```python
from build123d import *

# Parameters (mm, degrees)
SKETCH1_W           = 13
SKETCH1_H           = 1
SKETCH1_W_2         = 15
BOSS_EXTRUDE1_DEPTH = 6
BOSS_EXTRUDE2_DEPTH = 1


with BuildPart() as part:
    # Sketch1 → Boss-Extrude1 (new body)
    with BuildSketch(Plane(origin=(0, 0, 0), x_dir=(1, 0, 0), z_dir=(0, 1, 0))):
        with Locations((-9.5, 2.5)):
            Rectangle(SKETCH1_W, SKETCH1_H)
        Polygon((-17, 0), (-16, 0), (-16, 1), (-16, 2), (-16, 3), (-17, 3), align=None)
        with Locations((-8.5, 0.5)):
            Rectangle(SKETCH1_W_2, SKETCH1_H)
        Polygon((-1, 0), (0, 0), (0, 3), (-1, 3), (-1, 1), align=None)
    extrude(amount=BOSS_EXTRUDE1_DEPTH)

    # Sketch1_3 → Boss-Extrude2 (add)
    with BuildSketch(Plane(origin=(0, 0, 0), x_dir=(1, 0, 0), z_dir=(0, 1, 0))):
        Polygon((-16, 1), (-1, 1), (-1, 3), (-3, 3), (-3, 2), (-16, 2), align=None)
    extrude(amount=BOSS_EXTRUDE2_DEPTH)


solid = part.part
```
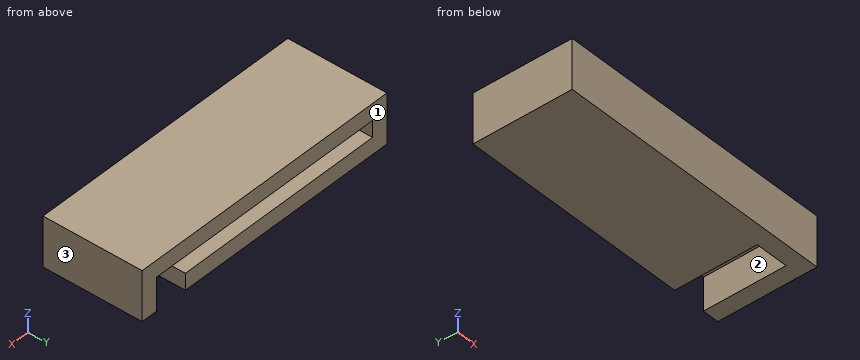
Read the model definition and answer for the solid it produces. Units are mm, in the model's axes. Face numbers are marked on the shaded views. Round coordinates to 2 decimals unless told otherwise and drop trailing zeros. Write each loop counter-clockwise with the first axis right and the second up, starting at its lowest first coordinate (ties: lowest second). Pieces come first, ordered by that corner, then holes. Notation, with made-up numbers: (61.5, 6) - (82.5, 6) arc R27 cw to (82.5, 27) - close; hole circle Ø10 at (-3.5, 25). An arc over 180 degrees is marked (long way). One line per item, written item: value.
Q1. For a pull along X with two mould halves and no side action, classify the marked faces 1, 2 and 3 as pulls with the +X half, pulls with the -X half, needs draft (parallel to the pull), parting line crosses it, or undercut.
The answers:
face 1: needs draft
face 2: undercut
face 3: pulls with the +X half
Q2. Find section C-C (x = -4.75). Determine the outline of the cut face in (y, z).
The answers:
outline: (0, -3) - (6, -3) - (6, -2) - (1, -2) - (1, -1) - (6, -1) - (6, 0) - (0, 0) - close
Q3. This flat-tipped pin is pushed along its axis until it touches: P1, Ø1.5, axis at y = 0.5, z = -0.5, coming from the +X side. Where does it stop, or does it pass through?
The answers:
P1: stops at x = 0
Q4. Find section A-A (z = -1.3). Determine the outline of the cut face in (x, y).
The answers:
outline: (-17, 0) - (0, 0) - (0, 6) - (-1, 6) - (-1, 1) - (-16, 1) - (-16, 6) - (-17, 6) - close
Q5. Find section B-B (y = 2). Determine the outline of the cut face in (x, z).
The answers:
outline: (-17, -3) - (-3, -3) - (-3, -2) - (-16, -2) - (-16, -1) - (-1, -1) - (-1, -3) - (0, -3) - (0, 0) - (-17, 0) - close
Q6. Straight lines are drawn through the part: line 1 (Z direction, x = -10.25, y = 2.9); line 2 (X direction, y = 1.3, z = -2.4); line 3 (X direction, y = 2.8, z = -1.05). For each, find the intervals that lie inside material, in ascending order. Write a range as from..to.
The answers:
line 1: z = -3..-2, -1..0
line 2: x = -17..-3, -1..0
line 3: x = -17..-16, -1..0
Q7. Find section D-D (x = -2.25). Determine the outline of the cut face in (y, z), and give its area (3 significant figures).
The answers:
outline: (0, -3) - (1, -3) - (1, -1) - (6, -1) - (6, 0) - (0, 0) - close
area: 8.00 mm2
